from build123d import *

# Parameters (mm, degrees)
F0_R     = 9.525
F1_DEPTH = 19.05
F0_R_2   = 12.7
F2_DEPTH = 38.1
F3_DEPTH = 50.8


with BuildPart() as f1:
    # F0 (on Top) → F1 (new body)
    with BuildSketch(Plane.XY):
        with BuildLine():
            Line((-60.325, -16.497784), (-22.225, -38.494829))
            ThreePointArc((-22.225, -38.494829), (0, -44.45), (22.225, -38.494829))
            Line((22.225, -38.494829), (60.325, -16.497784))
            ThreePointArc((60.325, -16.497784), (69.85, 0), (60.325, 16.497784))
            Line((60.325, 16.497784), (22.225, 38.494829))
            ThreePointArc((22.225, 38.494829), (0, 44.45), (-22.225, 38.494829))
            Line((-22.225, 38.494829), (-60.325, 16.497784))
            ThreePointArc((-60.325, 16.497784), (-69.85, 0), (-60.325, -16.497784))
        make_face()
        with Locations((-50.8, 0)):
            Circle(F0_R, mode=Mode.SUBTRACT)
        with BuildLine():
            ThreePointArc((34.342876, 6.35), (34.779164, 3.188313), (34.925, 0))
            ThreePointArc((34.925, 0), (34.779164, -3.188313), (34.342876, -6.35))
            ThreePointArc((34.342876, -6.35), (24.695704, -24.695704), (6.35, -34.342876))
            ThreePointArc((6.35, -34.342876), (0, -34.925), (-6.35, -34.342876))
            ThreePointArc((-6.35, -34.342876), (-24.695704, -24.695704), (-34.342876, -6.35))
            ThreePointArc((-34.342876, -6.35), (-34.925, 0), (-34.342876, 6.35))
            ThreePointArc((-34.342876, 6.35), (-24.695704, 24.695704), (-6.35, 34.342876))
            ThreePointArc((-6.35, 34.342876), (0, 34.925), (6.35, 34.342876))
            ThreePointArc((6.35, 34.342876), (24.695704, 24.695704), (34.342876, 6.35))
        make_face(mode=Mode.SUBTRACT)
        with Locations((50.8, 0)):
            Circle(F0_R, mode=Mode.SUBTRACT)
    extrude(amount=F1_DEPTH)

    # F0 (on Top) → F2 (join)
    with BuildSketch(Plane.XY):
        with BuildLine():
            ThreePointArc((25.4, 0), (25.197554, 3.200509), (24.593444, 6.35))
            ThreePointArc((24.593444, 6.35), (17.960512, 17.960512), (6.35, 24.593444))
            ThreePointArc((6.35, 24.593444), (0, 25.4), (-6.35, 24.593444))
            ThreePointArc((-6.35, 24.593444), (-17.960512, 17.960512), (-24.593444, 6.35))
            ThreePointArc((-24.593444, 6.35), (-25.4, 0), (-24.593444, -6.35))
            ThreePointArc((-24.593444, -6.35), (-17.960512, -17.960512), (-6.35, -24.593444))
            ThreePointArc((-6.35, -24.593444), (0, -25.4), (6.35, -24.593444))
            ThreePointArc((6.35, -24.593444), (17.960512, -17.960512), (24.593444, -6.35))
            ThreePointArc((24.593444, -6.35), (25.197554, -3.200509), (25.4, 0))
        make_face()
        Circle(F0_R_2, mode=Mode.SUBTRACT)
        with BuildLine():
            Line((-24.593444, 6.35), (-34.342876, 6.35))
            ThreePointArc((-34.342876, 6.35), (-34.925, 0), (-34.342876, -6.35))
            Line((-34.342876, -6.35), (-24.593444, -6.35))
            ThreePointArc((-24.593444, -6.35), (-25.4, 0), (-24.593444, 6.35))
        make_face()
        with BuildLine():
            Line((6.35, 24.593444), (6.35, 34.342876))
            ThreePointArc((6.35, 34.342876), (0, 34.925), (-6.35, 34.342876))
            Line((-6.35, 34.342876), (-6.35, 24.593444))
            ThreePointArc((-6.35, 24.593444), (0, 25.4), (6.35, 24.593444))
        make_face()
        with BuildLine():
            ThreePointArc((-6.35, -34.342876), (0, -34.925), (6.35, -34.342876))
            Line((6.35, -34.342876), (6.35, -24.593444))
            ThreePointArc((6.35, -24.593444), (0, -25.4), (-6.35, -24.593444))
            Line((-6.35, -24.593444), (-6.35, -34.342876))
        make_face()
        with BuildLine():
            ThreePointArc((34.342876, -6.35), (34.779164, -3.188313), (34.925, 0))
            ThreePointArc((34.925, 0), (34.779164, 3.188313), (34.342876, 6.35))
            Line((34.342876, 6.35), (24.593444, 6.35))
            ThreePointArc((24.593444, 6.35), (25.197554, 3.200509), (25.4, 0))
            ThreePointArc((25.4, 0), (25.197554, -3.200509), (24.593444, -6.35))
            Line((24.593444, -6.35), (34.342876, -6.35))
        make_face()
    extrude(amount=F2_DEPTH)

    # F0 (on Top) → F3 (join)
    with BuildSketch(Plane.XY):
        with BuildLine():
            Line((24.593444, 6.35), (34.342876, 6.35))
            ThreePointArc((34.342876, 6.35), (24.695704, 24.695704), (6.35, 34.342876))
            Line((6.35, 34.342876), (6.35, 24.593444))
            ThreePointArc((6.35, 24.593444), (17.960512, 17.960512), (24.593444, 6.35))
        make_face()
        with BuildLine():
            ThreePointArc((6.35, -34.342876), (24.695704, -24.695704), (34.342876, -6.35))
            Line((34.342876, -6.35), (24.593444, -6.35))
            ThreePointArc((24.593444, -6.35), (17.960512, -17.960512), (6.35, -24.593444))
            Line((6.35, -24.593444), (6.35, -34.342876))
        make_face()
        with BuildLine():
            ThreePointArc((-34.342876, -6.35), (-24.695704, -24.695704), (-6.35, -34.342876))
            Line((-6.35, -34.342876), (-6.35, -24.593444))
            ThreePointArc((-6.35, -24.593444), (-17.960512, -17.960512), (-24.593444, -6.35))
            Line((-24.593444, -6.35), (-34.342876, -6.35))
        make_face()
        with BuildLine():
            Line((-6.35, 24.593444), (-6.35, 34.342876))
            ThreePointArc((-6.35, 34.342876), (-24.695704, 24.695704), (-34.342876, 6.35))
            Line((-34.342876, 6.35), (-24.593444, 6.35))
            ThreePointArc((-24.593444, 6.35), (-17.960512, 17.960512), (-6.35, 24.593444))
        make_face()
    extrude(amount=F3_DEPTH)


solid = f1.part
Could you check a few things on this model? Use its own coordinates, in mm. A direction names the side the tool comes from. Coordinates: 2 decimals unless noted, no trailing zeros. Loops run counter-clockwise (first coordinate to the right, second up) from the corner with the lowest first, then second, coordinate; pieces in that order, holes last.
1. For faces 4 (the face through (-31.4, -16.3, 19.05)), 5 (the face through (30, -6.35, 44)), 6 (the face through (-6.35, 29, 44)), which set-ups out of +Z, -Z, +X, -X, +Y, -Y let a thin tool reach every point of the face, with its end or its side?
2. For P1, Ø5, axis at x = -32, z = 42.5, coming from the +Y side; P2, Ø4, axis at y = -31, z = 31.5, coming from the -X side; P3, Ø1.5, axis at y = 27, z = 8.5, coming from the -X side; P4, Ø11.5, axis at x = -50.8, y = 0, coming from the +Z side, each with a flat end and sliding along its axis, tell me the tip position at first contact or that it passes through.
3. Imagine slicing it at A-A (z = 21). Please give me the cut outline in (x, y) (3 decimals), and give its area (3 significant figures).
4. Imagine slicing it at D-D (x = 45.5). Please give me the cut outline in (y, z), and give its area (3 significant figures).
5. I need wall thicknesses on L1, parallel to Z at x = -45.5, y = 12; L2, parallel to Y at x = -6.5, z = 13.5; L3, parallel to Z at x = 26, y = -2. Which ranges of each line are inside material? Lowest first, please.
6. We'd pull the mould along Y, two halves only. Please class faces 1 (the face through (59.6, -3.65, 9.39)), 2 (the face through (20, 21, 50.8)), 3 (the face through (41.542, 27.342, 9.392)): released by +Y, released by -Y, zero draft, split by the parting line, or undercut.
7. Imagine slicing it at B-B (x = 0). Please give me the cut outline in (y, z) (3 decimals), and give its area (3 significant figures).
8. Imagine slicing it at C-C (y = 1.5). Please give me the cut outline in (x, z).
Computed values:
1. face 4: +Z
1. face 5: +Z, +X, -X
1. face 6: +Z, +Y, -Y
2. P1: stops at y = 18.7
2. P2: stops at x = -19.46
2. P3: stops at x = -43.43
2. P4: passes through
3. outline: (-34.343, -6.35) arc R34.925 ccw to (-6.35, -34.343) arc R34.925 ccw to (6.35, -34.343) arc R34.925 ccw to (34.343, -6.35) arc R34.925 ccw to (34.925, 0) arc R34.925 ccw to (34.343, 6.35) arc R34.925 ccw to (6.35, 34.343) arc R34.925 ccw to (-6.35, 34.343) arc R34.925 ccw to (-34.343, 6.35) arc R34.925 ccw to start; hole circle Ø25.4 at (0, 0)
3. area: 3,330 mm2
4. outline: (-25.06, 0) - (-7.91, 0) - (-7.91, 19.05) - (-25.06, 19.05) - close; (7.91, 0) - (25.06, 0) - (25.06, 19.05) - (7.91, 19.05) - close
4. area: 653 mm2
5. L1: z = 0 to 19.05
5. L2: y = -43.97 to -10.91, 10.91 to 43.97
5. L3: z = 0 to 38.1
6. face 1: undercut
6. face 2: zero draft
6. face 3: released by +Y
7. outline: (-44.45, 0) - (-12.7, 0) - (-12.7, 38.1) - (-34.925, 38.1) - (-34.925, 19.05) - (-44.45, 19.05) - close; (12.7, 0) - (44.45, 0) - (44.45, 19.05) - (34.925, 19.05) - (34.925, 38.1) - (12.7, 38.1) - close
7. area: 2,060 mm2
8. outline: (-69.79, 0) - (-60.21, 0) - (-60.21, 19.05) - (-69.79, 19.05) - close; (-41.39, 0) - (-12.61, 0) - (-12.61, 38.1) - (-34.89, 38.1) - (-34.89, 19.05) - (-41.39, 19.05) - close; (12.61, 0) - (41.39, 0) - (41.39, 19.05) - (34.89, 19.05) - (34.89, 38.1) - (12.61, 38.1) - close; (60.21, 0) - (69.79, 0) - (69.79, 19.05) - (60.21, 19.05) - close
